from build123d import *

# Parameters (mm, degrees)
MAIN_SHAPE_DEPTH                              = 6.35
FILLET1_R                                     = 3
ELBOW_X_MOUNT_HOLES_D                         = 1.9939
ELBOW_X_MOUNT_HOLES_DEPTH                     = 7.67
ELBOW_X_MOUNT_HOLES_TIP                       = 0.599027994
SKETCH6_W                                     = 23
SKETCH6_H                                     = 12
CUTOUT_FOR_WRIST_SERVO_DEPTH                  = 7.35
WRIST_SERVO_MOUNTING_HOLES_D                  = 1.9939
F_1_4_0_25_DIAMETER_HOLE_FOR_WRIST_DOWE_D     = 6.35
F_1_4_0_25_DIAMETER_HOLE_FOR_WRIST_DOWE_DEPTH = 18
F_1_4_0_25_DIAMETER_HOLE_FOR_WRIST_DOWE_TIP   = 1.907732465


with BuildPart() as part:
    # Sketch1 → main shape (new body)
    with BuildSketch(Plane.XY):
        Polygon((0, 17.159), (0, 30), (120, 30), (120, 0), (0, 0), (0, 12.841), (30, 12.841), (30, 17.159), align=None)
    extrude(amount=MAIN_SHAPE_DEPTH)

    # Fillet1
    fillet1_edges = [part.edges().sort_by_distance(p)[0] for p in [
        (0, 30, 3.175),
        (120, 30, 3.175),
        (120, 0, 3.175),
        (0, 0, 3.175),
    ]]
    fillet(fillet1_edges, radius=FILLET1_R)

    # elbow X mount holes
    with Locations(Plane.XY.offset(6.35)):
        with Locations((5, 26.625), (28.25, 26.625), (28.25, 3.375), (5, 3.375)):
            Hole(ELBOW_X_MOUNT_HOLES_D / 2, depth=ELBOW_X_MOUNT_HOLES_DEPTH)
            with Locations((0, 0, -(ELBOW_X_MOUNT_HOLES_DEPTH + ELBOW_X_MOUNT_HOLES_TIP / 2))):  # 118° drill point
                Cone(0, ELBOW_X_MOUNT_HOLES_D / 2, ELBOW_X_MOUNT_HOLES_TIP, mode=Mode.SUBTRACT)

    # Sketch6 → cutout for wrist servo (cut, through all)
    with BuildSketch(Plane.XY.offset(6.35)):
        with Locations((59, 15)):
            Rectangle(SKETCH6_W, SKETCH6_H)
    extrude(amount=-CUTOUT_FOR_WRIST_SERVO_DEPTH, mode=Mode.SUBTRACT)

    # wrist servo mounting holes (through all)
    with Locations(Plane.XY.offset(6.35)):
        with Locations((45, 15), (73, 15)):
            Hole(WRIST_SERVO_MOUNTING_HOLES_D / 2)

    # 1/4 (0.25) Diameter Hole (for wrist dowel)
    with Locations(Plane.XY.offset(6.35)):
        with Locations((105, 15)):
            Hole(F_1_4_0_25_DIAMETER_HOLE_FOR_WRIST_DOWE_D / 2, depth=F_1_4_0_25_DIAMETER_HOLE_FOR_WRIST_DOWE_DEPTH)
            with Locations((0, 0, -(F_1_4_0_25_DIAMETER_HOLE_FOR_WRIST_DOWE_DEPTH + F_1_4_0_25_DIAMETER_HOLE_FOR_WRIST_DOWE_TIP / 2))):  # 118° drill point
                Cone(0, F_1_4_0_25_DIAMETER_HOLE_FOR_WRIST_DOWE_D / 2, F_1_4_0_25_DIAMETER_HOLE_FOR_WRIST_DOWE_TIP, mode=Mode.SUBTRACT)


solid = part.part
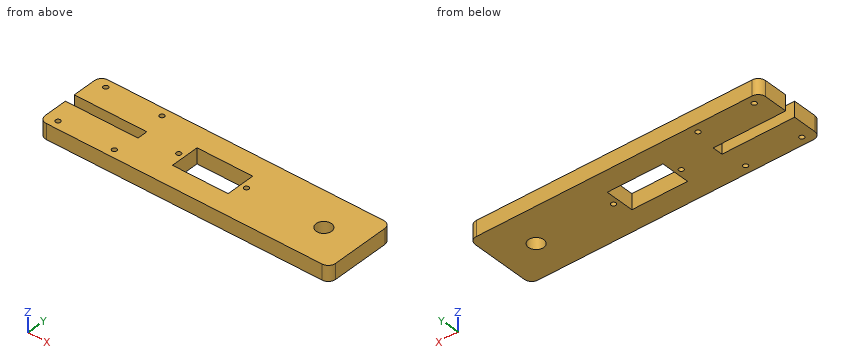
Build history of the part. All positions in model axes, mm. Give positions to 0.01 mm unless a question says otherwise; leave off trailing zeros. Loops run counter-clockwise (first coordinate to the right, second up) from the corner with the lowest first, then second, coordinate; pieces in that order, holes last. Notation, with made-up numbers: (-7.5, 61.25) -> (-3.5, 61.25) arc R13 ccw to (-3.5, 86.25) -> close; hole circle Ø6 at (4, 67.5). An arc over 180 degrees is marked (long way). Answer in a Markdown table with one row per item.
Item 1: Slice it at B-B on y = 10.5. Write the cut outline in (x, z).
Findings below:
| item | result |
|---|---|
| outline | (0, 0) -> (47.5, 0) -> (47.5, 6.35) -> (0, 6.35) -> close; (70.5, 0) -> (120, 0) -> (120, 6.35) -> (70.5, 6.35) -> close |
Item 2: Probe line 1 along X through (y, z) = (3.5, 5); line 2 along Y through (x, z) = (5, 5); line 3 along X through (y, z) = (11.75, 1.25). List the from-to ranges inside material, lowest first. Write a range as [from, to].
Findings below:
| item | result |
|---|---|
| line 1 | x = [0, 4.01], [5.99, 27.26], [29.24, 120] |
| line 2 | y = [0, 2.38], [4.37, 12.84], [17.16, 25.63], [27.62, 30] |
| line 3 | x = [0, 47.5], [70.5, 120] |
Item 3: Flat gauge pins, fed straight in: P1, Ø1.9, axis at y = 14, z = 2, coming from the -X side; P2, Ø2.5, axis at x = 5, y = 3.375, coming from the -Z side. Where does each tip first touch, or does it go through?
Findings below:
| item | result |
|---|---|
| P1 | stops at x = 30 |
| P2 | stops at z = 0 |
Item 4: Slice it at D-D on z = 3. Give the number of separate pieces and of enclosed holes in the cut face, plus the area to 3 significant figures.
Findings below:
| item | result |
|---|---|
| separate pieces | 1 |
| enclosed holes | 8 |
| area | 3,140 mm² |
Item 5: Slice it at A-A on x = 105. Write the cut outline in (y, z) (3 decimals).
Findings below:
| item | result |
|---|---|
| outline | (0, 0) -> (11.825, 0) -> (11.825, 6.35) -> (0, 6.35) -> close; (18.175, 0) -> (30, 0) -> (30, 6.35) -> (18.175, 6.35) -> close |
Item 6: Slice it at C-C on x = 28.25. Write the cut outline in (y, z).
Findings below:
| item | result |
|---|---|
| outline | (0, 0) -> (2.38, 0) -> (2.38, 6.35) -> (0, 6.35) -> close; (4.37, 0) -> (12.84, 0) -> (12.84, 6.35) -> (4.37, 6.35) -> close; (17.16, 0) -> (25.63, 0) -> (25.63, 6.35) -> (17.16, 6.35) -> close; (27.62, 0) -> (30, 0) -> (30, 6.35) -> (27.62, 6.35) -> close |
